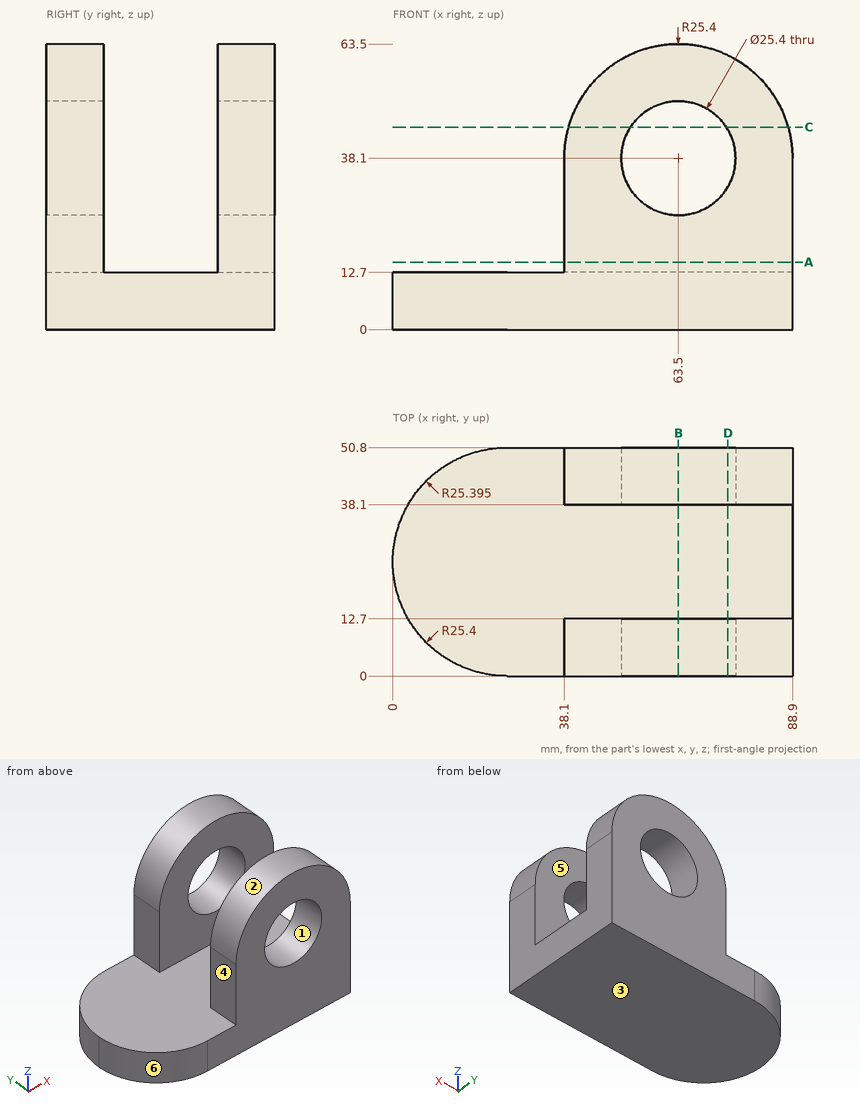
The figure shows three views and two pictorial views of one solid part (mm, origin at its lowest corner). Answer the questions. A direction names the side the tool comes from. Coordinates: 2 decimals unless noted, no trailing zeros. Loops run counter-clockwise (first coordinate to the right, second up) from the corner with the lowest first, then second, coordinate; pieces in that order, holes last. Notation, with made-up numbers: (62, 79) - (99, 79) arc R13 ccw to (99, 84) - close; hole circle Ø3 at (-28, -16.75). An arc over 180 degrees is marked (long way). Answer in a Markdown table with one row per item.
Q1. Find section A-A on z = 15. Write down the section's boundary in (x, y).
Here are the results:
| item | result |
|---|---|
| outline | (38.1, 0) - (88.9, 0) - (88.9, 12.7) - (38.1, 12.7) - close; (38.1, 38.1) - (88.9, 38.1) - (88.9, 50.8) - (38.1, 50.8) - close |
Q2. Find section C-C on z = 45. Write down the section's boundary in (x, y) (3 decimals).
Here are the results:
| item | result |
|---|---|
| outline | (39.055, 0) - (52.838, 0) - (52.838, 12.7) - (39.055, 12.7) - close; (39.055, 38.1) - (52.838, 38.1) - (52.838, 50.8) - (39.055, 50.8) - close; (74.162, 0) - (87.945, 0) - (87.945, 12.7) - (74.162, 12.7) - close; (74.162, 38.1) - (87.945, 38.1) - (87.945, 50.8) - (74.162, 50.8) - close |
Q3. Find section D-D on x = 74.5. Write down the section's boundary in (y, z), plus the area to 3 significant figures.
Here are the results:
| item | result |
|---|---|
| outline | (0, 0) - (50.8, 0) - (50.8, 31.75) - (38.1, 31.75) - (38.1, 12.7) - (12.7, 12.7) - (12.7, 31.75) - (0, 31.75) - close; (0, 44.45) - (12.7, 44.45) - (12.7, 60.99) - (0, 60.99) - close; (38.1, 44.45) - (50.8, 44.45) - (50.8, 60.99) - (38.1, 60.99) - close |
| area | 1,550 mm^2 |
Q4. Find section B-B on x = 63.5. Write down the section's boundary in (y, z), plus the area to 3 significant figures.
Here are the results:
| item | result |
|---|---|
| outline | (0, 0) - (50.8, 0) - (50.8, 25.4) - (38.1, 25.4) - (38.1, 12.7) - (12.7, 12.7) - (12.7, 25.4) - (0, 25.4) - close; (0, 50.8) - (12.7, 50.8) - (12.7, 63.5) - (0, 63.5) - close; (38.1, 50.8) - (50.8, 50.8) - (50.8, 63.5) - (38.1, 63.5) - close |
| area | 1,290 mm^2 |
Q5. For the marked faces 4, 5 and 6, determine the directions among +Z, -Z, +X, -X, +Y, -Y from which every point of the face is accessible in a straight line to the end or side of a thin tool.
Here are the results:
| item | result |
|---|---|
| face 4 | +Z, -X, +Y, -Y |
| face 5 | +Z, +X, -X |
| face 6 | +Z, -Z, -X, -Y |
Q6. Straight lines are drawn through the part: line 1 along Y through (x, z) = (44, 40.5); line 2 along Z through (x, y) = (63.5, 45.5); line 3 along X through (y, z) = (6, 38). For each, find the intervals that lie inside material, in ascending order. Write a range as [from, to].
Here are the results:
| item | result |
|---|---|
| line 1 | y = [0, 12.7], [38.1, 50.8] |
| line 2 | z = [0, 25.4], [50.8, 63.5] |
| line 3 | x = [38.1, 50.8], [76.2, 88.9] |
Q7. The mould has two halves that part along X. Classify the marked faces 1, 2 and 3: pulls with the +X half, pulls with the -X half, needs draft (parallel to the pull), parting line crosses it, or undercut.
Here are the results:
| item | result |
|---|---|
| face 1 | undercut |
| face 2 | parting line crosses it |
| face 3 | needs draft |
Q8. Given P1, Ø4, axis at x = 76, y = 10, coming from the +Z side; P2, Ø14, axis at y = 45, z = 31, coming from the -X side; P3, Ø1, axis at x = 50, y = 40.5, coming from the +Z side, each flat-ended and moving along its own axis, determine where each tip first touches the part or whether it passes through.
Here are the results:
| item | result |
|---|---|
| P1 | stops at z = 61.23 |
| P2 | stops at x = 38.1 |
| P3 | stops at z = 59.92 |
